```python
from build123d import *

# Parameters (mm, degrees)
ESQUISSE1_R             = 15
BASE_DEPTH              = 10
ESQUISSE2_R             = 2.5
ENL_V_MAT_EXTRU_1_DEPTH = 224.830292856


with BuildPart() as part:
    # Esquisse1 → BASE (new body)
    with BuildSketch(Plane(origin=(0, 0, 0), x_dir=(1, 0, 0), z_dir=(0, 1, 0))):
        Polygon((-100, 95), (-90, 95), (-90, 85), (-100, 85), (-100, -85), (-90, -85), (-90, -95), (-100, -95), (-100, -100), (-15, -100), (15, -100), (100, -100), (100, -95), (90, -95), (90, -85), (100, -85), (100, 85), (90, 85), (90, 95), (100, 95), (100, 100), (-100, 100), align=None)
        with Locations(Location((0, 0, 0), (0, 0, 270))):
            Circle(ESQUISSE1_R, mode=Mode.SUBTRACT)
    extrude(amount=BASE_DEPTH)

    # Esquisse2 → Enlèv. mat.-Extru.1 (cut, through all)
    with BuildSketch(Plane.XY.offset(100)):
        with Locations((-95, 5)):
            Circle(ESQUISSE2_R)
        with Locations(Location((95, 5, 0), (0, 0, 180))):
            Circle(ESQUISSE2_R)
    extrude(amount=-ENL_V_MAT_EXTRU_1_DEPTH, mode=Mode.SUBTRACT)


solid = part.part
```
Model file for the job. Use its own axes, mm. A direction names the side the tool comes from. Round coordinates to 2 decimals unless told otherwise and drop trailing zeros. Loops run counter-clockwise (first coordinate to the right, second up) from the corner with the lowest first, then second, coordinate; pieces in that order, holes last. Notation, with made-up numbers: M -2.5,9 L 8.5,9 A10 ccw 8.5,14 Z; hole C 63,38 d7. An arc over 180 degrees is marked long. Put each result on its own line as item: value. Start each with the question number.
Item 1: Cut at D-D (z = 0.5). List the corners of the cut face in (x, y), then the cut area to 3 significant figures.
Item 2: 3-axis set-ups, long thin cutter, end or side, ignore diameter. For faces 1 (the face through (1, 5, -100)), 2 (the face through (-93, 3, 95)), 3 (the face through (93, 3, 85)): which of +Z, -Z, +X, -X, +Y, -Y reach the whole face in a straight line?
Item 3: Drill centre lines: line 1 along X through (y, z) = (4.5, 0); line 2 along Y through (x, z) = (95, 96); line 3 along X through (y, z) = (6.5, -80.5). Where is each one in solid material? Low to high.
Item 4: Mould opens along X. For faces 4 (the face through (97.5, 4.9, -97.5)), 5 (the face through (90, 5, -90)), 6 (the face through (-1, 5, 100)) say: released by +X, released by -X, zero draft, split by the parting line, or undercut.
Item 5: Cut at A-A (x = -95). List the corners of the cut face in (y, z).
Item 6: Cut at B-B (x = 12). List the corners of the cut face in (y, z).
Item 7: Cut at C-C (y = 5). Give the number of separate pieces and of enclosed holes in the cut face, then the cut area to 3 significant figures.
Answer block:
1. outline: M -100,0 L -14.99,0 L -14.99,10 L -100,10 Z; M 14.99,0 L 100,0 L 100,10 L 14.99,10 Z; hole C -95,5 d5; hole C 95,5 d5
1. area: 1,660 mm2
2. face 1: -Z, +X, -X, +Y, -Y
2. face 2: -X, +Y, -Y
2. face 3: +X, +Y, -Y
3. line 1: -100 to -97.45, -92.55 to -15, 15 to 92.55, 97.45 to 100
3. line 2: 0 to 2.5, 7.5 to 10
3. line 3: -100 to -97, -93 to 93, 97 to 100
4. face 4: undercut
4. face 5: released by +X
4. face 6: zero draft
5. outline: M 0,-100 L 2.5,-100 L 2.5,-95 L 0,-95 Z; M 0,-85 L 2.5,-85 L 2.5,85 L 0,85 Z; M 0,95 L 2.5,95 L 2.5,100 L 0,100 Z; M 7.5,-100 L 10,-100 L 10,-95 L 7.5,-95 Z; M 7.5,-85 L 10,-85 L 10,85 L 7.5,85 Z; M 7.5,95 L 10,95 L 10,100 L 7.5,100 Z
6. outline: M 0,-100 L 10,-100 L 10,-9 L 0,-9 Z; M 0,9 L 10,9 L 10,100 L 0,100 Z
7. separate pieces: 7
7. enclosed holes: 1
7. area: 37,100 mm2
